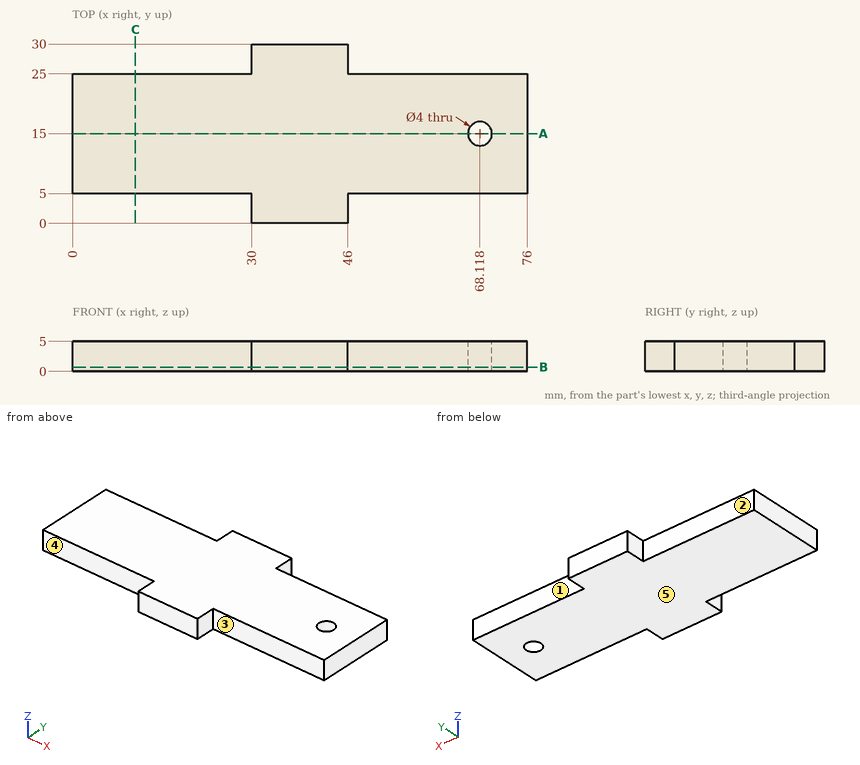
Geometry check sheet. Reference: drawing and pictorial views, mm from the part's lowest x, y, z. A direction names the side the tool comes from. Round coordinates to 2 decimals unless told otherwise and drop trailing zeros. Order: outer loops, then holes, each group sorted by start corner. A loop starts at its lowest first (then second) coordinate and runs counter-clockwise, first axis right, second up. Notation, with made-up numbers: M 65,-18 L 101,-18 A16 cw 101,0 Z; hole C -30.5,8.5 d1. An arc over 180 degrees is marked long. One line per item, written item: value. Start each with the question number.
1. Section check B-B on z = 0.7. Enter the section's corners in (x, y).
2. Scan lines: line 1 along X through (y, z) = (27.25, 0.65); line 2 along Y through (x, z) = (52, 1.7); line 3 along Y through (x, z) = (69, 2.2) (1 decimal). Record each from-to range of solid material in increasing order.
3. Section check C-C on x = 10.5. Enter the section's corners in (y, z), and give its area (3 significant figures).
4. Gauge pin test, flat ends, axial feed: P1, Ø2.5, axis at x = 14.5, z = 3, coming from the -Y side; P2, Ø2.5, axis at x = 11.5, z = 2.5, coming from the +Y side; P3, Ø3.5, axis at x = 68.12, y = 15, coming from the +Z side; P4, Ø2.5, axis at y = 2.5, z = 3.5, coming from the -X side. Record the tip position at first contact, or that the pin passes through.
5. Access from +Z, -Z, +X, -X, +Y, -Y to the whole of each face (thin tool, end or side, straight path). Record for the marked faces 1, 2, 3, 4 and 5.
6. Section check A-A on y = 15. Enter the section's corners in (x, z), and give its area (3 significant figures).
Results found:
1. outline: M 0,5 L 30,5 L 30,0 L 46,0 L 46,5 L 76,5 L 76,25 L 46,25 L 46,30 L 30,30 L 30,25 L 0,25 Z; hole C 68.12,15 d4
2. line 1: 30 to 46
2. line 2: 5 to 25
2. line 3: 5 to 13.2, 16.8 to 25
3. outline: M 5,0 L 25,0 L 25,5 L 5,5 Z
3. area: 100 mm^2
4. P1: y = 5
4. P2: y = 25
4. P3: through
4. P4: x = 30
5. face 1: +Z, -Z, +X, +Y
5. face 2: +Z, -Z, -X, +Y
5. face 3: +Z, -Z, +X, -Y
5. face 4: +Z, -Z, -X, -Y
5. face 5: -Z, +X, -X, +Y, -Y
6. outline: M 0,0 L 66.12,0 L 66.12,5 L 0,5 Z; M 70.12,0 L 76,0 L 76,5 L 70.12,5 Z
6. area: 360 mm^2
